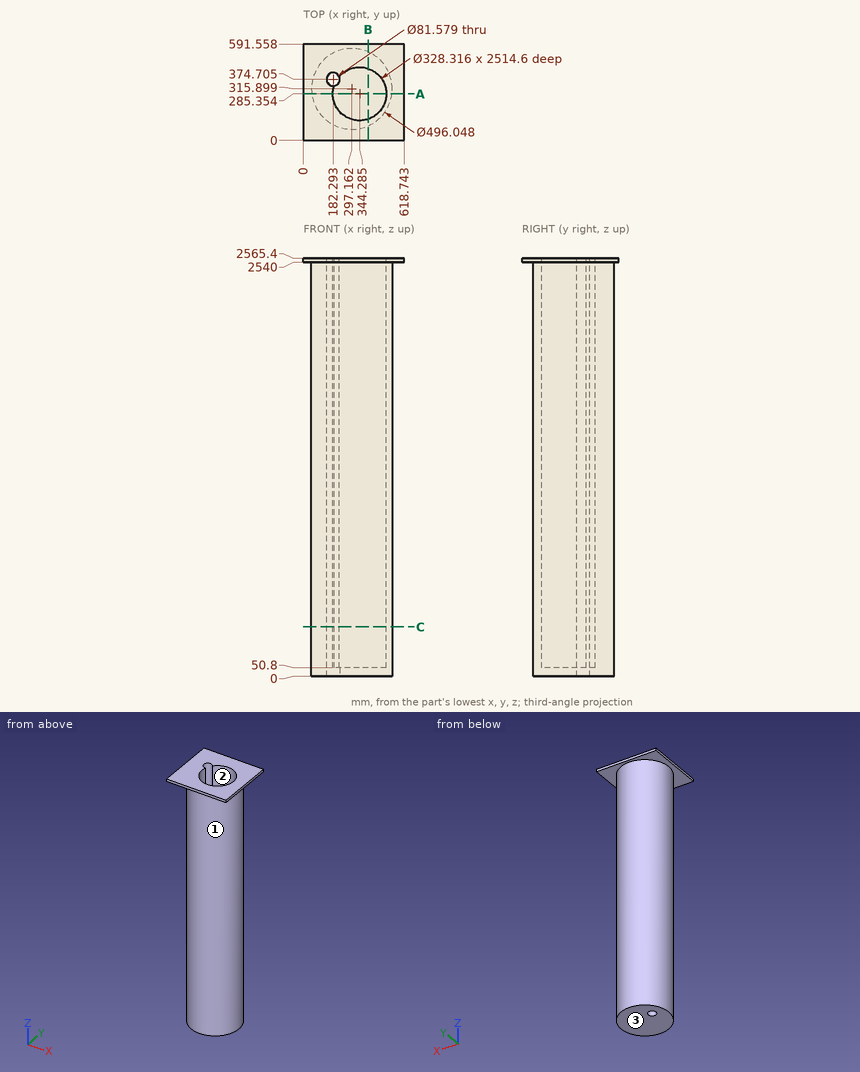
Answer from the drawing. Dimensions are ordinates in mm from the lowest x, y and z of the part. Give positions to 0.01 mm unless a question says otherwise; leave off trailing zeros. Write each loop counter-clockwise with the first axis right and the second up, starting at its lowest first coordinate (ties: lowest second). Pieces come first, ordered by that corner, then holes.
1) For a pull along Y with two mould halves and no side action, classify the marked faces 1, 2 and 3 as pulls with the +Y half, pulls with the -Y half, needs draft (parallel to the pull), parting line crosses it, or undercut.
2) Section B-B (x = 397.5) is taken. Write down the section's boundary in (y, z), and give its area (3 significant figures).
3) Given P1, Ø3, axis at y = 515.5, z = 1405, coming from the -X side (1 decimal); P2, Ø8, axis at y = 61, z = 2174.5, coming from the -X side; P3, Ø6, axis at y = 415.5, z = 644, coming from the -X side; P4, Ø2, axis at x = 211, z = 937.5, coming from the -Y side (1 decimal), each flat-ended and moving along its own axis, determine where each tip first touches the part or whether it passes through.
4) Section C-C (z = 302) is taken. Write down the section's boundary in (x, y) (1 decimal).
5) Find the intervals of material crossed by L1, parallel to Z at x = 580.5, y = 103.5; L2, parallel to Z at x = 368, y = 341; L3, parallel to Y at x = 321.5, z = 1749.5 (1 decimal), in increasing order.
6) Section A-A (y = 285.5) is taken. Write down the section's boundary in (x, z), and give its area (3 significant figures).
Response:
1. face 1: parting line crosses it
1. face 2: undercut
1. face 3: needs draft
2. outline: (0, 2540) - (89.08, 2540) - (89.08, 0) - (542.72, 0) - (542.72, 2540) - (591.56, 2540) - (591.56, 2565.4) - (440.65, 2565.4) - (440.65, 50.8) - (130.06, 50.8) - (130.06, 2565.4) - (0, 2565.4) - close
2. area: 386,000 mm2
3. P1: stops at x = 147.9
3. P2: passes through
3. P3: stops at x = 68.72
3. P4: stops at y = 83
4. outline: circle Ø496 at (297.2, 315.9); hole (187.6, 334.3) arc R164.2 ccw (long way) to (219.3, 391.8) arc R40.8 ccw (long way) to start
5. L1: z = 2540 to 2565.4
5. L2: z = 0 to 50.8
5. L3: y = 69.1 to 122.8, 447.9 to 562.7
6. outline: (0, 2540) - (51.01, 2540) - (51.01, 0) - (543.32, 0) - (543.32, 2540) - (618.74, 2540) - (618.74, 2565.4) - (508.44, 2565.4) - (508.44, 50.8) - (180.13, 50.8) - (180.13, 2565.4) - (0, 2565.4) - close
6. area: 441,000 mm2
